The model under review builds one solid part; all positions refer to its coordinate system, in mm. Face numbers are marked on the shaded views. Coordinates: 2 decimals unless noted, no trailing zeros. Loops run counter-clockwise (first coordinate to the right, second up) from the corner with the lowest first, then second, coordinate; pieces in that order, holes last. Notation, with made-up numbers: M -20,21.25 L 25,21.25 A34 ccw 25,58.25 Z; hole C 57.25,25 d7. An arc over 180 degrees is marked long. Use one line per item in the form item = value.
```python
from build123d import *

# Parameters (mm, degrees)
SKETCH2_R          = 1.5
CUT_EXTRUDE1_DEPTH = 10
CIRPATTERN1_COUNT  = 4


with BuildPart() as part:
    # Sketch1 → Revolve1 (revolve)
    with BuildSketch(Plane(origin=(0, 0, 0), x_dir=(1, 0, 0), z_dir=(0, 1, 0)), mode=Mode.PRIVATE) as revolve1_sk:
        with BuildLine():
            Line((-33.620030864, 40.5), (-47.2, 40.5))
            ThreePointArc((-47.2, 40.5), (-51.796194078, 42.403805922), (-53.7, 47))
            Line((-53.7, 47), (-53.7, 47.5))
            Line((-53.7, 47.5), (-53.7, 47.7))
            Line((-53.7, 47.7), (-54, 47.7))
            Line((-54, 47.7), (-54, 49.5))
            Line((-54, 49.5), (-54, 60.5))
            Line((-54, 60.5), (-55.7, 60.5))
            Line((-55.7, 60.5), (-55.7, 47))
            ThreePointArc((-55.7, 47), (-53.21040764, 40.98959236), (-47.2, 38.5))
            Line((-47.2, 38.5), (-31.890858754, 38.5))
            ThreePointArc((-31.890858754, 38.5), (-26.327846361, 32.743886889), (-24.3, 25))
            Line((-24.3, 25), (-23.3, 25))
            ThreePointArc((-23.3, 25), (-26.116018423, 34.310652999), (-33.620030864, 40.5))
        make_face()
    revolve(revolve1_sk.sketch.rotate(Axis((0, 0, 0), (0, 0, -1)), 180), axis=Axis((0, 0, 0), (0, 0, -1)))

    # Sketch2 → Cut-Extrude1 (cut)
    with BuildSketch(Plane(origin=(0, 55.7, 0), x_dir=(1, 0, 0), z_dir=(0, 1, 0))):
        with Locations(Location((0, 57.5, 0), (0, 0, 270))):
            Circle(SKETCH2_R)
    cut_extrude1 = extrude(amount=-CUT_EXTRUDE1_DEPTH, mode=Mode.SUBTRACT)

    # CirPattern1: Cut-Extrude1 ×4 about axis
    cirpattern1_axis = Axis((0, 0, 0), (0, 0, 1))
    for i in range(1, CIRPATTERN1_COUNT):
        add(cut_extrude1.rotate(cirpattern1_axis, i * 360 / CIRPATTERN1_COUNT), mode=Mode.SUBTRACT)

    # Sketch4 → Revolve2 (revolve)
    with BuildSketch(Plane(origin=(0, 0, 0), x_dir=(1, 0, 0), z_dir=(0, 1, 0)), mode=Mode.PRIVATE) as revolve2_sk:
        with BuildLine():
            Line((-24.3, 25), (-23.3, 25))
            ThreePointArc((-23.3, 25), (-25.812155139, 11.590644472), (-33.007896924, 0))
            Line((-33.007896924, 0), (-34.379125514, 0))
            ThreePointArc((-34.379125514, 0), (-26.914612018, 11.522344685), (-24.3, 25))
        make_face()
    revolve(revolve2_sk.sketch.rotate(Axis((0, 0, 0), (0, 0, -1)), 180), axis=Axis((0, 0, 0), (0, 0, -1)))

    # Sketch12 → Cut-Revolve2 (revolve, cut)
    with BuildSketch(Plane(origin=(0, 0, 0), x_dir=(0, 0, -1), z_dir=(1, 0, 0)), mode=Mode.PRIVATE) as cut_revolve2_sk:
        Polygon((0.171963045, 34.804821283), (0.171963045, 32.977261807), (-3.294935837, 32.977261807), align=None)
    revolve(cut_revolve2_sk.sketch.rotate(Axis((0, 0, 33.840895414), (0, 0, -1)), 90), axis=Axis((0, 0, 33.840895414), (0, 0, -1)), mode=Mode.SUBTRACT)


solid = part.part
```
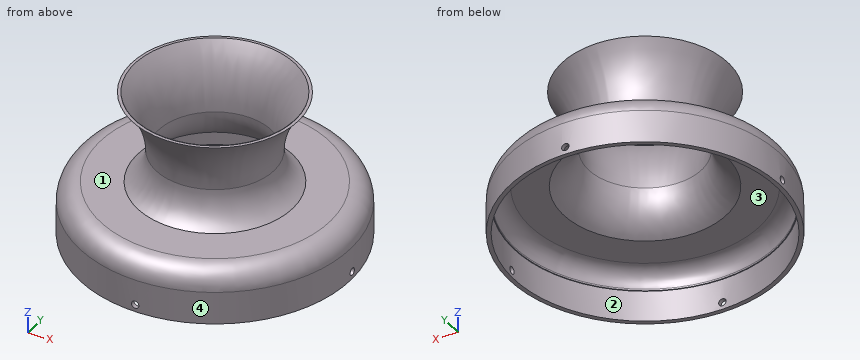
1. Add section B-B (x = 0). Count the separate pieces of the cut face and the enclosed holes in it, then the cut area to 3 significant figures.
Response values:
separate_pieces = 4
enclosed_holes = 0
area = 232 mm^2
2. Insertion check: P1, Ø5, axis at x = -23.5, y = -39.5, coming from the +Z side; P2, Ø6, axis at x = 15, z = -49, coming from the +Y side; P3, Ø8, axis at y = -26.5, z = -24.5, coming from the -X side. Each pin has a flat end and moves straight along its axis. Give the tip position at first contact, or say it passes through.
Response values:
P1 = -38.5
P2 = 54.39
P3 = -9.19
3. Add section A-A (z = -57.5). State the section outline as (x, y) points, then the cut area to 3 significant figures.
Response values:
outline = M -55.68,-1.5 A55.7 ccw -1.5,-55.68 L -1.5,-53.98 A54 cw -53.98,-1.5 Z; M -55.68,1.5 L -53.98,1.5 A54 cw -1.5,53.98 L -1.5,55.68 A55.7 ccw Z; M 1.5,-55.68 A55.7 ccw 55.68,-1.5 L 53.98,-1.5 A54 cw 1.5,-53.98 Z; M 1.5,53.98 A54 cw 53.98,1.5 L 55.68,1.5 A55.7 ccw 1.5,55.68 Z
area = 565 mm^2
4. The part is to be moulded in two halves that separate along Y. For the marked faces 1, 2, 3 and 4, say which applies: pulls with the +Y half, pulls with the -Y half, needs draft (parallel to the pull), parting line crosses it, or undercut.
Response values:
face_1 = needs draft
face_2 = undercut
face_3 = undercut
face_4 = parting line crosses it
5. Add section D-D (z = -8). State the section outline as (x, y) points.
Response values:
outline = C 0,0 d57.12; hole C 0,0 d54.86
6. Wall thickness on line 1 along Y through (x, z) = (0, -51); line 2 along Z through (x, y) = (-29.5, 2.5); line 3 along Z through (x, y) = (-33, 14): over which ranges is each line inside the solid? List them lowest first. Write a range as from..to.
Response values:
line_1 = -55.7..-54, 54..55.7
line_2 = -38.12..-36.81, -6.18..-4.33
line_3 = -40.5..-38.5
